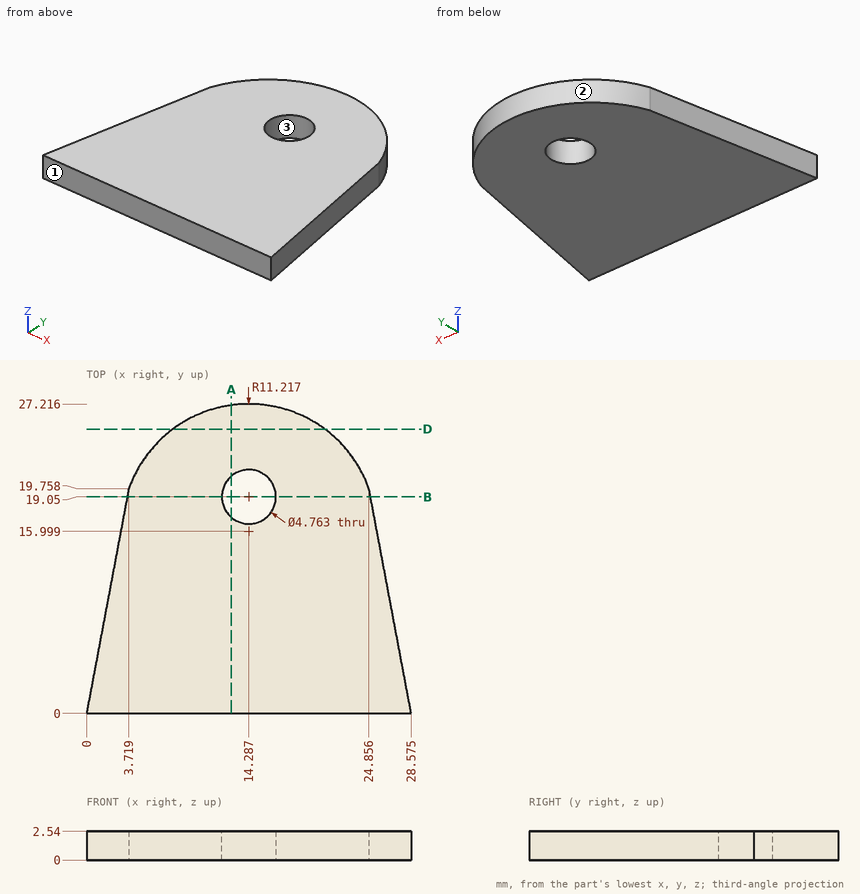
Verification items for this drawing (mm, ordinates from the low corner). Round coordinates to 2 decimals unless told otherwise and drop trailing zeros. Loops run counter-clockwise (first coordinate to the right, second up) from the corner with the lowest first, then second, coordinate; pieces in that order, holes last. Notation, with made-up numbers: (10, 48.5) -> (64, 48.5) arc R33 ccw to (64, 84.5) -> close; hole circle Ø3 at (0.25, 12.25). An arc over 180 degrees is marked (long way). Answer in a Markdown table with one row per item.
Q1. Sectioned sample at D-D on y = 25. Enter the section's corners in (x, z).
Data:
| item | result |
|---|---|
| outline | (7.59, 0) -> (20.98, 0) -> (20.98, 2.54) -> (7.59, 2.54) -> close |
Q2. Sectioned sample at A-A on x = 12.75. Enter the section's corners in (y, z).
Data:
| item | result |
|---|---|
| outline | (0, 0) -> (17.23, 0) -> (17.23, 2.54) -> (0, 2.54) -> close; (20.87, 0) -> (27.11, 0) -> (27.11, 2.54) -> (20.87, 2.54) -> close |
Q3. Thickness scan on L1, parallel to Y at x = 16, z = 2.15 (1 decimal); L2, parallel to Y at x = 19.5, z = 0.3; L3, parallel to Y at x = 21.75, z = 2.2 (1 decimal). Record the ranges inside material, lowest first.
Data:
| item | result |
|---|---|
| L1 | y = 0 to 17.4, 20.7 to 27.1 |
| L2 | y = 0 to 25.93 |
| L3 | y = 0 to 24.4 |
Q4. Release check for a two-part mould opening along X. For the marked faces 1, 2 and 3 record: released by +X, released by -X, zero draft, split by the parting line, or undercut.
Data:
| item | result |
|---|---|
| face 1 | zero draft |
| face 2 | split by the parting line |
| face 3 | undercut |
Q5. Go/stop test with flat-tipped pins: P1, Ø1, axis at y = 11, z = 0.5, coming from the -X side; P2, Ø5, axis at x = 24, y = 5, coming from the -Z side; P3, Ø1, axis at y = 13.5, z = 1.5, coming from the -X side. Record where each tip stops, or that it passes through.
Data:
| item | result |
|---|---|
| P1 | stops at x = 1.98 |
| P2 | stops at z = 0 |
| P3 | stops at x = 2.45 |
Q6. Sectioned sample at B-B on y = 19.05. Enter the section's corners in (x, z) (1 decimal).
Data:
| item | result |
|---|---|
| outline | (3.6, 0) -> (11.9, 0) -> (11.9, 2.5) -> (3.6, 2.5) -> close; (16.7, 0) -> (25, 0) -> (25, 2.5) -> (16.7, 2.5) -> close |
